Here's how the part is built. I have some questions about the finished solid (model axes, mm). Face numbers are marked on the shaded views. Coordinates: 2 decimals unless noted, no trailing zeros. Write each loop counter-clockwise with the first axis right and the second up, starting at its lowest first coordinate (ties: lowest second). Pieces come first, ordered by that corner, then holes.
(1) Please list where these lines run through material, in increasing order: probe 1 along Y at (x, z) = (0, 12.9); probe 2 along Z at (x, y) = (15.5, 6.5); probe 3 along Y at (x, z) = (-11, 13).
(2) Imagine slicing it at D-D, the plane z = 3.25. List the corners of the cut face in (x, y) for me, plus the area to 3 significant figures.
(3) For pin 1 Ø8 at (x, z) = (-3.5, 5.5) entering from +Y; pin 2 Ø2 at (x, y) = (3.5, -2.5) entering from +Z; pin 3 Ø5 at (y, z) = (-9.5, 2) entering from +X, each with a flat end and sliding along its axis, tell me the tip position at first contact or that it passes through.
(4) Imagine slicing it at A-A, the plane y = 0. List the corners of the cut face in (x, z) for me.
(5) Thinking about a two-plate mould opening in X: for the marked faces 1, 2 and 3, which applies, released by +X, released by -X, zero draft, split by the parting line, or undercut?
(6) Imagine slicing it at B-B, the plane z = 13.25. List the corners of the cut face in (x, y) for me.
```python
from build123d import *

# Parameters (mm, degrees)
F0_R     = 21
F1_DEPTH = 12
F2_R     = 23
F2_R_2   = 21
F3_DEPTH = 16
F4_SIZE  = 1


with BuildPart() as f1:
    # F0 (on Top) → F1 (new body)
    with BuildSketch(Plane.XY):
        Circle(F0_R)
    extrude(amount=F1_DEPTH)

    # F2 (on Top) → F3 (join)
    with BuildSketch(Plane.XY):
        Circle(F2_R)
        Circle(F2_R_2, mode=Mode.SUBTRACT)
    extrude(amount=F3_DEPTH)

    # F4
    f4_edges = [f1.edges().sort_by_distance(p)[0] for p in [
        (-21, 0, 16),
    ]]
    chamfer(f4_edges, length=F4_SIZE)


solid = f1.part
```
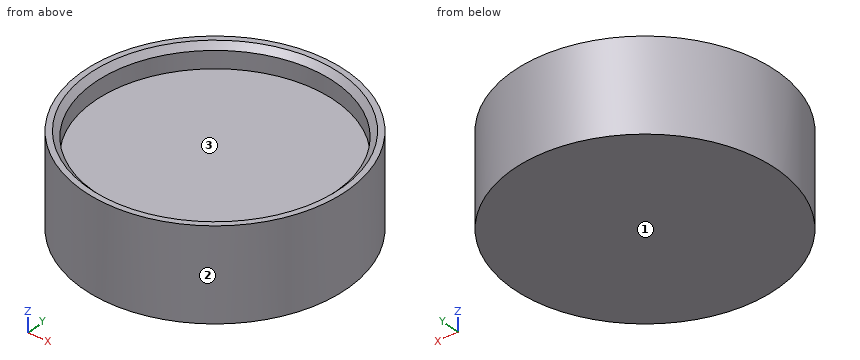
Recorded:
1. probe 1: y = -23 to -21, 21 to 23
1. probe 2: z = 0 to 12
1. probe 3: y = -20.2 to -17.89, 17.89 to 20.2
2. outline: circle Ø46 at (0, 0)
2. area: 1,660 mm2
3. pin 1: stops at y = 23
3. pin 2: stops at z = 12
3. pin 3: stops at x = 21.91
4. outline: (-23, 0) - (23, 0) - (23, 16) - (22, 16) - (21, 15) - (21, 12) - (-21, 12) - (-21, 15) - (-22, 16) - (-23, 16) - close
5. face 1: zero draft
5. face 2: split by the parting line
5. face 3: undercut
6. outline: circle Ø46 at (0, 0); hole circle Ø42 at (0, 0)
